Could you check a few things on this model? Use its own coordinates, in mm. A direction names the side the tool comes from. Coordinates: 2 decimals unless noted, no trailing zeros. Write each loop counter-clockwise with the first axis right and the second up, starting at its lowest first coordinate (ties: lowest second). Pieces come first, ordered by that corner, then holes.
Item 1: For P1, Ø5, axis at y = -1.5, z = 19.5, coming from the -X side; P2, Ø4, axis at y = -17, z = 19.5, coming from the -X side; P3, Ø7, axis at y = 50.5, z = 19, coming from the -X side; P4, Ø4.5, axis at x = 16, y = -52.07, coming from the +Z side, each with a flat end and sliding along its axis, tell me the tip position at first contact or that it passes through.
Item 2: I want a section at B-B on z = 26.5. Please give me the cut outline in (x, y).
Item 3: I want a section at D-D on x = 8. Please give me the cut outline in (y, z), then the cut area to 3 significant figures.
Item 4: Which directions (+Z, -Z, +X, -X, +Y, -Y) give clear straight access to the entire face, cutting with the end or side of a thin tool? Please do faces 1 (the cylindrical face through (13.952, -35.981, 15.776)), 2 (the flat face through (40, 0, 16)).
Item 5: I want a section at C-C on x = 16. Please give me the cut outline in (y, z), then the cut area to 3 significant figures.
Item 6: Thinking about a two-plate mould opening in Y: for faces 3 (the flat face through (26.4, 32.74, 15.78)), 4 (the flat face through (0, 52, 16)), 5 (the cylindrical face through (-0.444, -38.072, 15.776)), 6 (the flat face through (20, 25, 16)), which applies, +Y half, -Y half, draft (parallel to the pull), parting line (faces both ways), or undercut?
Item 7: I want a section at A-A on x = 28. Please give me the cut outline in (y, z), then the cut area to 3 significant figures.
Item 8: If I drill on probe 1 along Y at (x, z) = (8.5, 6.5); probe 2 along Y at (x, z) = (8, 10); probe 3 along Y at (x, z) = (16, 17), over which ranges is the centre line in solid material (lowest first)?
from build123d import *

# Parameters (mm, degrees)
SKETCH1_R           = 2.05
BOSS_EXTRUDE2_DEPTH = 32


with BuildPart() as part:
    # Sketch1 → Boss-Extrude2 (new body)
    with BuildSketch(Plane.XY):
        with BuildLine():
            Line((40, -5), (14.464466094, -30.535533906))
            ThreePointArc((14.464466094, -30.535533906), (-2.606601718, -54.67766953), (21.535533906, -37.606601718))
            Line((21.535533906, -37.606601718), (52.071067812, -7.071067812))
            Line((52.071067812, -7.071067812), (52.071067812, 7.071067812))
            Line((52.071067812, 7.071067812), (0, 59.142135624))
            Line((0, 59.142135624), (0, 45))
            Line((0, 45), (40, 5))
            Line((40, 5), (40, -5))
        make_face()
        with Locations((0, -52.071067812)):
            Circle(SKETCH1_R, mode=Mode.SUBTRACT)
        with Locations((16, -52.071067812)):
            Circle(SKETCH1_R, mode=Mode.SUBTRACT)
        with Locations((16, -36.071067812)):
            Circle(SKETCH1_R, mode=Mode.SUBTRACT)
        with Locations((0, -36.071067812)):
            Circle(SKETCH1_R, mode=Mode.SUBTRACT)
        with Locations((8, 44.071067812)):
            Circle(SKETCH1_R, mode=Mode.SUBTRACT)
    extrude(amount=BOSS_EXTRUDE2_DEPTH)


solid = part.part
Response values:
1. P1: stops at x = 40
1. P2: stops at x = 26
1. P3: stops at x = 0
1. P4: stops at z = 32
2. outline: (0, 45) - (40, 5) - (40, -5) - (14.46, -30.54) arc R15 ccw (long way) to (21.54, -37.61) - (52.07, -7.07) - (52.07, 7.07) - (0, 59.14) - close; hole circle Ø4.1 at (0, -52.07); hole circle Ø4.1 at (0, -36.07); hole circle Ø4.1 at (8, 44.07); hole circle Ø4.1 at (16, -52.07); hole circle Ø4.1 at (16, -36.07)
3. outline: (-59.07, 0) - (-29.07, 0) - (-29.07, 32) - (-59.07, 32) - close; (37, 0) - (42.02, 0) - (42.02, 32) - (37, 32) - close; (46.12, 0) - (51.14, 0) - (51.14, 32) - (46.12, 32) - close
3. area: 1,280 mm2
4. face 1: +Z, -Z
4. face 2: +Z, -Z, -X
5. outline: (-56.76, 0) - (-54.12, 0) - (-54.12, 32) - (-56.76, 32) - close; (-50.02, 0) - (-38.12, 0) - (-38.12, 32) - (-50.02, 32) - close; (-34.02, 0) - (-29, 0) - (-29, 32) - (-34.02, 32) - close; (29, 0) - (43.14, 0) - (43.14, 32) - (29, 32) - close
5. area: 1,080 mm2
6. face 3: +Y half
6. face 4: draft
6. face 5: undercut
6. face 6: undercut
7. outline: (-31.14, 0) - (-17, 0) - (-17, 32) - (-31.14, 32) - close; (17, 0) - (31.14, 0) - (31.14, 32) - (17, 32) - close
7. area: 905 mm2
8. probe 1: y = -59.06 to -29.08, 36.5 to 42.08, 46.06 to 50.64
8. probe 2: y = -59.07 to -29.07, 37 to 42.02, 46.12 to 51.14
8. probe 3: y = -56.76 to -54.12, -50.02 to -38.12, -34.02 to -29, 29 to 43.14
